Input: part model. Units: mm. Frame: model coordinates. A direction names the side the tool comes from. Coordinates: 2 decimals unless noted, no trailing zeros. Order: outer loops, then holes, each group sorted by start corner. A loop starts at its lowest first (then second) coordinate and runs counter-clockwise, first axis right, second up. Notation, with made-up numbers: (29, 8.5) -> (50, 8.5) arc R16 cw to (50, 30.5) -> close; hole circle Ø5 at (36, 22.25). An arc over 180 degrees is marked (long way). Write each question's results on one line, items separated by ' | '.
```python
from build123d import *

# Parameters (mm, degrees)
SKETCH002_W     = 50
SKETCH002_H     = 25
PAD_DEPTH       = 3
SKETCH003_R     = 8
SKETCH003_R_2   = 1.3
POCKET_DEPTH    = 3.001
SKETCH004_W     = 16
SKETCH004_H     = 20
POCKET001_DEPTH = 3.001
SKETCH_W        = 15
SKETCH_H        = 37
PAD001_DEPTH    = 3
SKETCH001_R     = 1.25
POCKET002_DEPTH = 3.001


with BuildPart() as part:
    # Sketch002 → Pad (new body)
    with BuildSketch(Plane.YZ):
        with Locations((17.5, 9.5)):
            Rectangle(SKETCH002_W, SKETCH002_H)
    extrude(amount=-PAD_DEPTH)

    # Sketch003 → Pocket (cut, through all)
    with BuildSketch(Plane.YZ):
        with Locations((4.5, 10)):
            Circle(SKETCH003_R)
        with Locations((30.5, 10)):
            Circle(SKETCH003_R)
        with Locations((-3.5, 19)):
            Circle(SKETCH003_R_2)
        with Locations((38.5, 19)):
            Circle(SKETCH003_R_2)
        with Locations((38.5, 1.5)):
            Circle(SKETCH003_R_2)
        with Locations((-3.5, 1.5)):
            Circle(SKETCH003_R_2)
    extrude(amount=-POCKET_DEPTH, mode=Mode.SUBTRACT)

    # Sketch004 → Pocket001 (cut, through all)
    with BuildSketch(Plane.YZ):
        with Locations((17.5, 10)):
            Rectangle(SKETCH004_W, SKETCH004_H)
    extrude(amount=-POCKET001_DEPTH, mode=Mode.SUBTRACT)

    # Sketch → Pad001 (join)
    with BuildSketch(Plane.XY):
        with Locations((7.5, 18.5)):
            Rectangle(SKETCH_W, SKETCH_H)
    extrude(amount=-PAD001_DEPTH)

    # Sketch001 → Pocket002 (cut, through all)
    with BuildSketch(Plane.XY):
        with Locations((10, 23.5)):
            Circle(SKETCH001_R)
        with Locations((10, 13.5)):
            Circle(SKETCH001_R)
    extrude(amount=-POCKET002_DEPTH, mode=Mode.SUBTRACT)


solid = part.part
```
(1) Mould query, pull axis Z, two halves, no side actions, for faces 4 (the face through (-1, 42.5, 9)), 5 (the face through (-1, 9.5, 18)), 6 (the face through (-1, 17, 22)), 7 (the face through (-1.48, 37.2, 1.56)). Classes: +Z half, -Z half, draft (parallel to the pull), parting line (faces both ways), or undercut.
Return value:
face 4: draft | face 5: undercut | face 6: +Z half | face 7: undercut
(2) Cut plane C-C, the plane z = 10. Return loops of the section in (x, y), plus the area to 3 significant figures.
Return value:
outline: (-3, -7.5) -> (0, -7.5) -> (0, -3.5) -> (-3, -3.5) -> close; (-3, 38.5) -> (0, 38.5) -> (0, 42.5) -> (-3, 42.5) -> close | area: 24.0 mm2
(3) Cut plane D-D, the plane y = -4. Return loops of the section in (x, z), plus the area to 3 significant figures.
Return value:
outline: (-3, -3) -> (0, -3) -> (0, 0.3) -> (-3, 0.3) -> close; (-3, 2.7) -> (0, 2.7) -> (0, 17.8) -> (-3, 17.8) -> close; (-3, 20.2) -> (0, 20.2) -> (0, 22) -> (-3, 22) -> close | area: 60.6 mm2
(4) Reachability of faces 1 (the face through (7, 37, -1)), 2 (the face through (-1, 25.5, 2)), 3 (the face through (8.75, 23.55, -1.48)) from +Z, -Z, +X, -X, +Y, -Y: full face, straight path, thin tool, end or side. Return the list, or none.
Return value:
face 1: +Z, -Z, +X, +Y | face 2: +X, -X | face 3: +Z, -Z
(5) Line query: line 1 along Y through (x, z) = (10, -1.45); line 2 along Z through (x, y) = (-2.15, 4.5); line 3 along Z through (x, y) = (3, 31). Output: solid intervals per line, ascending. Write a range as from..to.
Return value:
line 1: 0..12.25, 14.75..22.25, 24.75..37 | line 2: -3..2, 18..22 | line 3: -3..0
(6) Cut plane B-B, the plane y = 20.5. Return loops of the section in (x, z).
Return value:
outline: (-3, -3) -> (15, -3) -> (15, 0) -> (-3, 0) -> close; (-3, 20) -> (0, 20) -> (0, 22) -> (-3, 22) -> close
(7) Pin query (flat end, axial travel): P1, Ø10, axis at y = 29, z = 15, coming from the -X side; P2, Ø9, axis at x = 10, y = 22, coming from the +Z side; P3, Ø3.5, axis at x = 8.5, z = -1, coming from the -Y side; P4, Ø2.5, axis at x = 8.5, z = -1.5, coming from the +Y side. Return the tip coordinate at first contact, or that it passes through.
Return value:
P1: x = -3 | P2: z = 0 | P3: y = 0 | P4: y = 37
(8) Cut plane A-A, the plane z = 19. Return loops of the section in (x, y), plus the area to 3 significant figures.
Return value:
outline: (-3, -7.5) -> (0, -7.5) -> (0, -4.8) -> (-3, -4.8) -> close; (-3, -2.2) -> (0, -2.2) -> (0, 9.5) -> (-3, 9.5) -> close; (-3, 25.5) -> (0, 25.5) -> (0, 37.2) -> (-3, 37.2) -> close; (-3, 39.8) -> (0, 39.8) -> (0, 42.5) -> (-3, 42.5) -> close | area: 86.4 mm2
